Check sheet for the drawn part. Datum: minimum x, y, z corner. Units: mm. A direction names the side the tool comes from. Round coordinates to 2 decimals unless told otherwise and drop trailing zeros. Write each loop counter-clockwise with the first axis right and the second up, starting at its lowest first coordinate (ties: lowest second). Pieces come first, ordered by that corner, then holes.
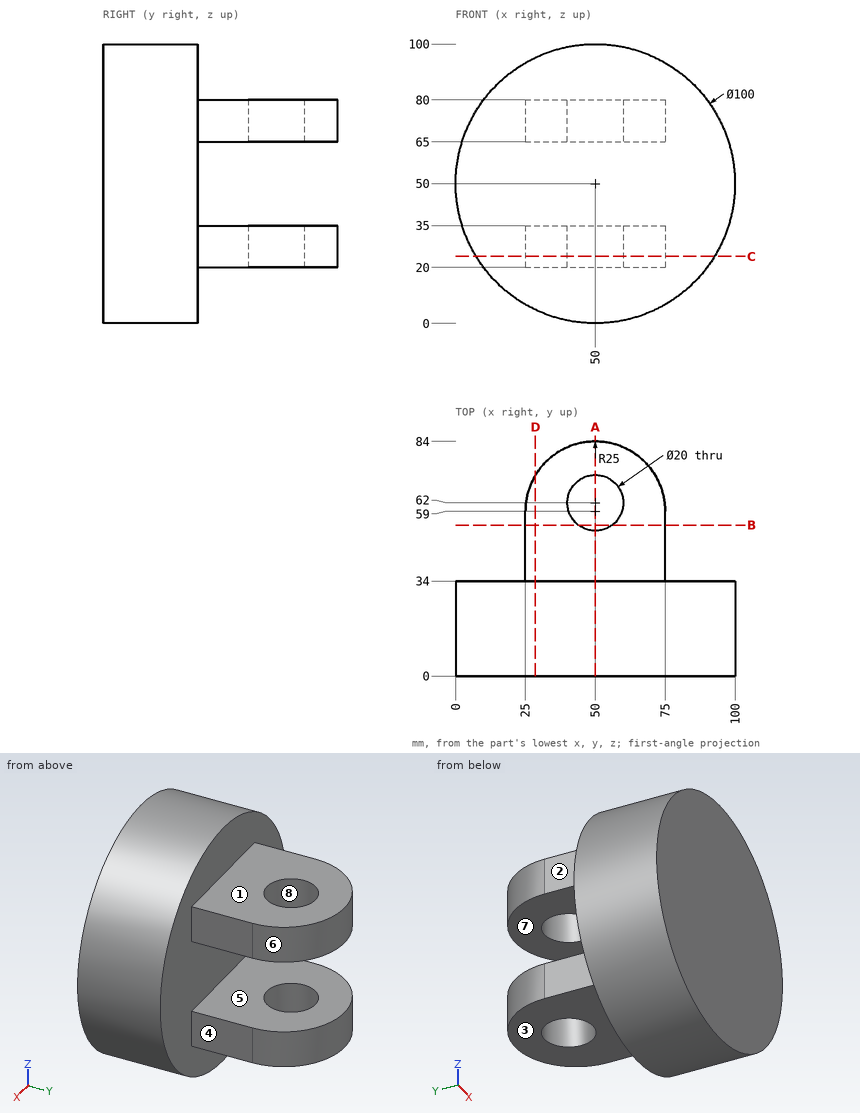
Q1. Material ranges on line 1 along Z through (x, y) = (67.5, 49); line 2 along Y through (x, z) = (50, 70); line 3 along Y through (x, z) = (36, 15), recorded low to high.
Recorded:
line 1: z = 20 to 35, 65 to 80
line 2: y = 0 to 52, 72 to 84
line 3: y = 0 to 34
Q2. Depth check by flat-ended pin: P1, Ø3, axis at x = 45.5, y = 54, coming from the +Z side; P2, Ø7.5, axis at y = 48, z = 28.5, coming from the -X side; P3, Ø12, axis at y = 52, z = 29.5, coming from the +X side; P4, Ø12, axis at x = 12, z = 70, coming from the -Y side. Enter the tip coordinate at first touch or a pass-through.
Recorded:
P1: stops at z = 80
P2: stops at x = 25
P3: stops at x = 75
P4: stops at y = 0
Q3. Sectioned sample at A-A (x = 50). Enter the section's corners in (y, z), plus the area to 3 significant figures.
Recorded:
outline: (0, 0) - (34, 0) - (34, 20) - (52, 20) - (52, 35) - (34, 35) - (34, 65) - (52, 65) - (52, 80) - (34, 80) - (34, 100) - (0, 100) - close; (72, 20) - (84, 20) - (84, 35) - (72, 35) - close; (72, 65) - (84, 65) - (84, 80) - (72, 80) - close
area: 4,300 mm2
Q4. Release check for a two-part mould opening along X. For the marked faces 6, 7 and 8 record: released by +X, released by -X, zero draft, split by the parting line, or undercut.
Recorded:
face 6: split by the parting line
face 7: zero draft
face 8: undercut
Q5. Sectioned sample at C-C (z = 24). Enter the section's corners in (x, y), plus the area to 3 significant figures.
Recorded:
outline: (7.29, 0) - (92.71, 0) - (92.71, 34) - (75, 34) - (75, 59) arc R25 ccw to (25, 59) - (25, 34) - (7.29, 34) - close; hole circle Ø20 at (50, 62)
area: 4,820 mm2
Q6. Sectioned sample at D-D (x = 28.5). Enter the section's corners in (y, z).
Recorded:
outline: (0, 4.86) - (34, 4.86) - (34, 20) - (71.76, 20) - (71.76, 35) - (34, 35) - (34, 65) - (71.76, 65) - (71.76, 80) - (34, 80) - (34, 95.14) - (0, 95.14) - close
Q7. Tool access check on the marked faces 1, 2, 3, 4 and 5. Record the directions out of +Z, -Z, +X, -X, +Y, -Y that give a thin tool (end or side, any length) a straight path to the whole face; none if there is none.
Recorded:
face 1: +Z, +X, -X, +Y
face 2: +Z, -Z, -X, +Y
face 3: -Z, +X, -X, +Y
face 4: +Z, -Z, +X, +Y
face 5: +X, -X, +Y
Q8. Sectioned sample at B-B (y = 54). Enter the section's corners in (x, z).
Recorded:
outline: (25, 20) - (44, 20) - (44, 35) - (25, 35) - close; (25, 65) - (44, 65) - (44, 80) - (25, 80) - close; (56, 20) - (75, 20) - (75, 35) - (56, 35) - close; (56, 65) - (75, 65) - (75, 80) - (56, 80) - close
